Read the model definition and answer for the solid it produces. Units are mm, in the model's axes. Face numbers are marked on the shaded views. A direction names the side the tool comes from. Give positions to 0.01 mm unless a question says otherwise; leave off trailing zeros. Order: outer loops, then holes, each group sorted by start corner. A loop starts at its lowest first (then second) coordinate and runs counter-clockwise, first axis right, second up. Notation, with made-up numbers: M -37.5,39 L -5.5,39 A12 cw -5.5,58 Z; hole C -2,59.25 d2. An arc over 180 degrees is marked long. One line per item, written item: value. Start each with the question number.
from build123d import *

# Parameters (mm, degrees)
SKETCH1_W           = 25
SKETCH1_H           = 52
BOSS_EXTRUDE1_DEPTH = 2
SKETCH2_W           = 25
SKETCH2_H           = 25
BOSS_EXTRUDE2_DEPTH = 2
SKETCH3_W           = 25
SKETCH3_H           = 25
BOSS_EXTRUDE3_DEPTH = 2
SKETCH5_R           = 4
CUT_EXTRUDE2_DEPTH  = 21
SKETCH7_R           = 2.5
CUT_EXTRUDE4_DEPTH  = 84
SKETCH8_R           = 2
CUT_EXTRUDE5_DEPTH  = 10


with BuildPart() as part:
    # Sketch1 → Boss-Extrude1 (new body)
    with BuildSketch(Plane.XY):
        with Locations((-0.174770451, 4.502942624)):
            Rectangle(SKETCH1_W, SKETCH1_H)
    extrude(amount=BOSS_EXTRUDE1_DEPTH)

    # Sketch2 → Boss-Extrude2 (add)
    with BuildSketch(Plane(origin=(0, 30.502942624, 0), x_dir=(1, 0, 0), z_dir=(0, 1, 0))):
        with Locations((-0.174770451, -12.5)):
            Rectangle(SKETCH2_W, SKETCH2_H)
    extrude(amount=BOSS_EXTRUDE2_DEPTH)

    # Sketch3 → Boss-Extrude3 (add)
    with BuildSketch(Plane(origin=(0, -21.497057376, 0), x_dir=(-1, 0, 0), z_dir=(0, -1, 0))):
        with Locations((0.174770451, -12.5)):
            Rectangle(SKETCH3_W, SKETCH3_H)
    extrude(amount=BOSS_EXTRUDE3_DEPTH)

    # Sketch5 → Cut-Extrude2 (cut)
    with BuildSketch(Plane(origin=(0, 0, 0), x_dir=(-1, 0, 0), z_dir=(0, 0, -1))):
        with Locations((0.174770451, 4.502942624)):
            Circle(SKETCH5_R)
    extrude(amount=-CUT_EXTRUDE2_DEPTH, mode=Mode.SUBTRACT)

    # Sketch7 → Cut-Extrude4 (cut)
    with BuildSketch(Plane(origin=(0, -23.497057376, 0), x_dir=(-1, 0, 0), z_dir=(0, -1, 0))):
        with Locations(Location((0.174770451, -20, 0), (0, 0, 90))):
            Circle(SKETCH7_R)
    extrude(amount=-CUT_EXTRUDE4_DEPTH, mode=Mode.SUBTRACT)

    # Sketch8 → Cut-Extrude5 (cut)
    with BuildSketch(Plane(origin=(0, 0, 0), x_dir=(-1, 0, 0), z_dir=(0, 0, -1))):
        with Locations((5.174770451, -19.497057376)):
            Circle(SKETCH8_R)
        with Locations((-4.825229549, -19.497057376)):
            Circle(SKETCH8_R)
        with Locations((-4.825229549, 28.502942624)):
            Circle(SKETCH8_R)
        with Locations((5.174770451, 28.502942624)):
            Circle(SKETCH8_R)
    extrude(amount=-CUT_EXTRUDE5_DEPTH, mode=Mode.SUBTRACT)


solid = part.part
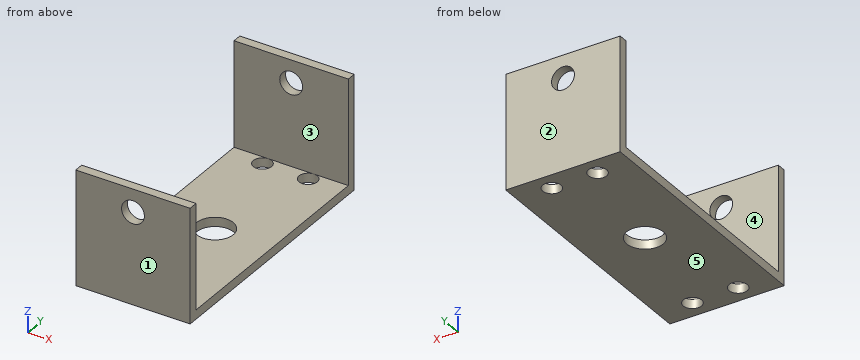
Q1. Consider probe 1 along Y at (x, z) = (9, 20.75); probe 2 along Y at (x, z) = (4, 1.75); probe 3 along X at (y, z) = (-22.8, 20). Determine where each line is inside the solid, lowest interval first.
Q2. Find section C-C, the plane y = 2.5. Give the vertices of the cut face in (x, z), then the cut area to 3 significant figures.
Q3. Each of these flat-tipped pins is pushed along its axis until it touches: pin 1 (4 mm diameter, centred on x = -6.5, y = -5.5, fed in from +Z); pin 2 (4.5 mm diameter, centred on x = 4.83, y = 28.5, fed in from +Z); pin 3 (6.5 mm diameter, centred on x = -0.17, y = 4.5, fed in from -Z). Where does it stop, or does it pass through?
Q4. Determine the mould class of the marked faces 1, 2 and 3 for opening direction Y: released by +Y, released by -Y, zero draft, split by the parting line, or undercut.
Q5. A tool of negligible diameter and unlimited length cuts with its end or side. For the marked faces 4 and 5, from which of +Z, -Z, +X, -X, +Y, -Y can it reach the whole face along a straight path? Write none if from no direction.
Q6. Find section B-B, the plane z = 11.25. Give the vertices of the cut face in (x, y), then the cut area to 3 significant figures.
Q7. Find section D-D, the plane x = 10.75. Give the vertices of the cut face in (y, z), then the cut area to 3 significant figures.
Q8. Find section A-A, the plane z = 20. Give the vertices of the cut face in (x, y), then the cut area to 3 significant figures.
Evaluation:
1. probe 1: -23.5 to -21.5, 30.5 to 32.5
1. probe 2: -23.5 to -21.32, -17.68 to 26.68, 30.32 to 32.5
1. probe 3: -12.67 to -2.67, 2.33 to 12.33
2. outline: M -12.67,0 L -3.64,0 L -3.64,2 L -12.67,2 Z; M 3.29,0 L 12.33,0 L 12.33,2 L 3.29,2 Z
2. area: 36.2 mm2
3. pin 1: z = 2
3. pin 2: z = 25
3. pin 3: through
4. face 1: released by -Y
4. face 2: released by +Y
4. face 3: undercut
5. face 4: +Z, +X, -X
5. face 5: -Z, +X, -X, +Y, -Y
6. outline: M -12.67,-23.5 L 12.33,-23.5 L 12.33,-21.5 L -12.67,-21.5 Z; M -12.67,30.5 L 12.33,30.5 L 12.33,32.5 L -12.67,32.5 Z
6. area: 100 mm2
7. outline: M -23.5,0 L 32.5,0 L 32.5,25 L 30.5,25 L 30.5,2 L -21.5,2 L -21.5,25 L -23.5,25 Z
7. area: 204 mm2
8. outline: M -12.67,-23.5 L -2.67,-23.5 L -2.67,-21.5 L -12.67,-21.5 Z; M -12.67,30.5 L -2.67,30.5 L -2.67,32.5 L -12.67,32.5 Z; M 2.33,-23.5 L 12.33,-23.5 L 12.33,-21.5 L 2.33,-21.5 Z; M 2.33,30.5 L 12.33,30.5 L 12.33,32.5 L 2.33,32.5 Z
8. area: 80.0 mm2
